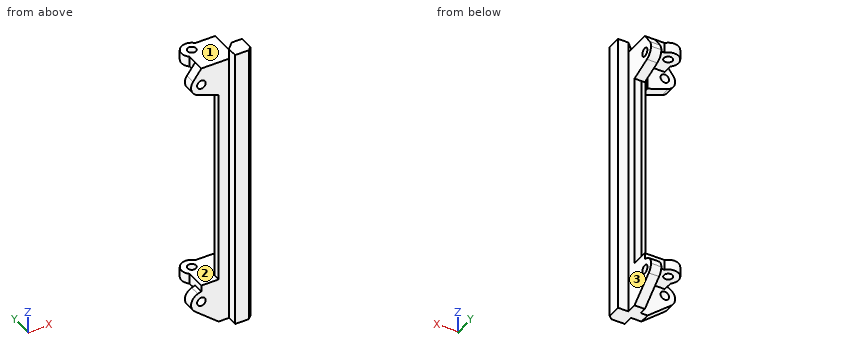
from build123d import *

# Parameters (mm, degrees)
F1_DEPTH  = 80
F2_R      = 1.25
F3_DEPTH  = 3
F4_DEPTH  = 3
F5_R      = 1.25
F6_DEPTH  = 3
F7_R      = 1.25
F8_DEPTH  = 3
F9_SIZE   = 1
F10_R     = 1.25
F10_W     = 3
F10_H     = 13
F11_DEPTH = 3
F12_W     = 3
F12_H     = 13
F12_R     = 1.25
F13_DEPTH = 3
F14_W     = 8
F14_H     = 3
F14_W_2   = 2
F15_DEPTH = 10
F17_DEPTH = 3
F16_R     = 1.25
F18_DEPTH = 25


with BuildPart() as f1:
    # F0 (on Top) → F1 (new body)
    with BuildSketch(Plane.XY):
        Polygon((40, 3), (40, 0), (45, 0), (45, 5), (42, 5), (42, 8), (40, 8), (40, 5), (37, 5), (37, 3), align=None)
    extrude(amount=F1_DEPTH)

    # F2 (on face) → F3 (join)
    with BuildSketch(Plane.XY.offset(80)):
        with BuildLine():
            Line((32, 3), (37, 3))
            Line((37, 3), (37, 5))
            Line((37, 5), (40, 5))
            Line((40, 5), (40, 8))
            Line((40, 8), (42, 8))
            Line((42, 8), (42, 13))
            Line((42, 13), (36.2360679775, 13))
            ThreePointArc((36.2360679775, 13), (36.8025170769, 12.0704662693), (37, 11))
            ThreePointArc((37, 11), (35.2247448714, 8.2613872125), (32, 8.7639320225))
            Line((32, 8.7639320225), (32, 3))
        make_face()
        with BuildLine():
            ThreePointArc((36.2360679775, 13), (31.8786796564, 13.1213203436), (32, 8.7639320225))
            ThreePointArc((32, 8.7639320225), (35.2247448714, 8.2613872125), (37, 11))
            ThreePointArc((37, 11), (36.8025170769, 12.0704662693), (36.2360679775, 13))
        make_face()
        with Locations((34, 11)):
            Circle(F2_R, mode=Mode.SUBTRACT)
    extrude(amount=-F3_DEPTH)

    # F2 (on face) → F4 (join)
    with BuildSketch(Plane.XY.offset(80)):
        Polygon((42, 5), (40, 3), (40, 0), (45, 0), (45, 5), align=None)
    extrude(amount=F4_DEPTH)

    # F5 (on face) → F6 (join)
    with BuildSketch(Plane.XZ.offset(-3)):
        with BuildLine():
            Line((32, 77), (32, 78))
            ThreePointArc((32, 78), (30.6583592135, 77.683281573), (29.6, 76.8))
            ThreePointArc((29.6, 76.8), (29.1245100257, 74.144688707), (30.97393957, 72.1809221376))
            ThreePointArc((30.97393957, 72.1809221376), (33.7207293091, 72.5425438671), (35, 75))
            ThreePointArc((35, 75), (34.8025170769, 76.0704662693), (34.2360679775, 77))
            Line((34.2360679775, 77), (32, 77))
        make_face()
        with Locations((32, 75)):
            Circle(F5_R, mode=Mode.SUBTRACT)
        with BuildLine():
            ThreePointArc((29.6, 76.8), (30.6583592135, 77.683281573), (32, 78))
            Line((32, 78), (32, 80))
            Line((32, 80), (29.6, 76.8))
        make_face()
        with BuildLine():
            Line((37, 77), (34.2360679775, 77))
            ThreePointArc((34.2360679775, 77), (34.8025170769, 76.0704662693), (35, 75))
            ThreePointArc((35, 75), (33.7207293091, 72.5425438671), (30.97393957, 72.1809221376))
            Line((30.97393957, 72.1809221376), (37, 69.9876155112))
            Line((37, 69.9876155112), (37, 77))
        make_face()
    extrude(amount=-F6_DEPTH)

    # F7 (on face) → F8 (join)
    with BuildSketch(Plane.YZ.offset(42)):
        with BuildLine():
            Line((8, 69.9876155112), (14.02606043, 72.1809221376))
            ThreePointArc((14.02606043, 72.1809221376), (10.5156676094, 73.3183066353), (10.7639320225, 77))
            Line((10.7639320225, 77), (8, 77))
            Line((8, 77), (8, 69.9876155112))
        make_face()
        with BuildLine():
            ThreePointArc((14.02606043, 72.1809221376), (15.4574561329, 73.2792706909), (16, 75))
            ThreePointArc((16, 75), (15.8460498942, 75.9486832981), (15.4, 76.8))
            ThreePointArc((15.4, 76.8), (14.3416407865, 77.683281573), (13, 78))
            Line((13, 78), (13, 77))
            Line((13, 77), (10.7639320225, 77))
            ThreePointArc((10.7639320225, 77), (10.5156676094, 73.3183066353), (14.02606043, 72.1809221376))
        make_face()
        with Locations((13, 75)):
            Circle(F7_R, mode=Mode.SUBTRACT)
        with BuildLine():
            ThreePointArc((13, 78), (14.3416407865, 77.683281573), (15.4, 76.8))
            Line((15.4, 76.8), (13, 80))
            Line((13, 80), (13, 78))
        make_face()
    extrude(amount=-F8_DEPTH)

    # F9
    f9_edges = [f1.edges().sort_by_distance(p)[0] for p in [
        (45, 0, 41.5),
    ]]
    chamfer(f9_edges, length=F9_SIZE)

    # F10 (on face) → F11 (join)
    with BuildSketch(Plane.XZ.offset(-3)):
        with BuildLine():
            ThreePointArc((30.0936794849, 5.6835496781), (33.2808275557, 5.2871637033), (35, 8))
            ThreePointArc((35, 8), (33.7229608507, 10.4558920796), (30.9790627288, 10.8209372712))
            ThreePointArc((30.9790627288, 10.8209372712), (29.0435836969, 8.5095121614), (30.0936794849, 5.6835496781))
        make_face()
        with Locations((32, 8)):
            Circle(F10_R, mode=Mode.SUBTRACT)
        with BuildLine():
            ThreePointArc((30.9790627288, 10.8209372712), (33.7229608507, 10.4558920796), (35, 8))
            ThreePointArc((35, 8), (33.2808275557, 5.2871637033), (30.0936794849, 5.6835496781))
            Line((30.0936794849, 5.6835496781), (37, 0))
            Line((37, 0), (37, 13))
            Line((37, 13), (30.9790627288, 10.8209372712))
        make_face()
        with Locations((38.5, 6.5)):
            Rectangle(F10_W, F10_H)
    extrude(amount=-F11_DEPTH)

    # F12 (on face) → F13 (join)
    with BuildSketch(Plane.YZ.offset(42)):
        with Locations((6.5, 6.5)):
            Rectangle(F12_W, F12_H)
        with BuildLine():
            ThreePointArc((14.9063205151, 5.6835496781), (10.0435836969, 7.4904878386), (14.0209372712, 10.8209372712))
            Line((14.0209372712, 10.8209372712), (8, 13))
            Line((8, 13), (8, 0))
            Line((8, 0), (14.9063205151, 5.6835496781))
        make_face()
        with BuildLine():
            ThreePointArc((14.9063205151, 5.6835496781), (15.7128362967, 6.7191724443), (16, 8))
            ThreePointArc((16, 8), (15.4558920796, 9.7229608507), (14.0209372712, 10.8209372712))
            ThreePointArc((14.0209372712, 10.8209372712), (10.0435836969, 7.4904878386), (14.9063205151, 5.6835496781))
        make_face()
        with Locations((13, 8)):
            Circle(F12_R, mode=Mode.SUBTRACT)
    extrude(amount=-F13_DEPTH)

    # F14 (on face) → F15 (join)
    with BuildSketch(Plane.XZ.offset(-3)):
        with Locations((36, 11.5)):
            Rectangle(F14_W, F14_H)
        with Locations((41, 11.5)):
            Rectangle(F14_W_2, F14_H)
    extrude(amount=-F15_DEPTH)

    # F16 (on face) → F17 (join)
    with BuildSketch(Plane.XY.offset(13)):
        with BuildLine():
            Line((32, 13), (36.2360679775, 13))
            ThreePointArc((36.2360679775, 13), (31.8786796564, 13.1213203436), (32, 8.7639320225))
            Line((32, 8.7639320225), (32, 13))
        make_face()
    extrude(amount=-F17_DEPTH)

    # F16 (on face) → F18 (cut)
    with BuildSketch(Plane.XY.offset(13)):
        with Locations((34, 11)):
            Circle(F16_R)
    extrude(amount=-F18_DEPTH, mode=Mode.SUBTRACT)


solid = f1.part
Could you check a few things on this model? Use its own coordinates, in mm. Face numbers are marked on the shaded views. Coordinates: 2 decimals unless noted, no trailing zeros. Write each loop counter-clockwise with the first axis right and the second up, starting at its lowest first coordinate (ties: lowest second). Pieces come first, ordered by that corner, then holes. Notation, with made-up numbers: M -36.75,-34 L 9.25,-34 A10 cw 9.25,-25 Z; hole C -26.75,47.25 d7. An arc over 180 degrees is marked long. One line per question, with ' | ' between items.
1) If we mould it in two halves opening along Z, with no side actions, what happens to the marked faces 1, 2 and 3? For each: released by +Z, released by -Z, zero draft, split by the parting line, or undercut.
Checks:
face 1: released by +Z | face 2: undercut | face 3: zero draft
2) For pin 1 Ø9 at (y, z) = (11.5, 76.5) entering from -X; pin 2 Ø3 at (y, z) = (7.5, 51) entering from -X; pin 3 Ø0.8 at (y, z) = (5.5, 73) entering from +X, each with a flat end and sliding along its axis, tell me the tip position at first contact or that it passes through.
Checks:
pin 1: x = 31 | pin 2: x = 40 | pin 3: x = 42
3) Imagine slicing it at A-A, the plane z = 37.5. Write out the boundary of the cut face in (x, y).
Checks:
outline: M 37,3 L 40,3 L 40,0 L 44,0 L 45,1 L 45,5 L 42,5 L 42,8 L 40,8 L 40,5 L 37,5 Z
4) I need wall thicknesses on probe 1 along Y at (x, z) = (34, 78.4); probe 2 along Z at (x, y) = (31.75, 12); probe 3 along Y at (x, z) = (40.55, 75). Which ranges of each line are inside material? Lowest first, please. Write a range as [from, to].
Checks:
probe 1: [3, 9.75], [12.25, 14] | probe 2: [10, 13], [77, 80] | probe 3: [0, 11.75], [14.25, 16]
5) Imagine slicing it at B-B, the plane y = 11. Write out the boundary of the cut face in (x, z), and give its area (3 significant figures).
Checks:
outline: M 31,10 L 32.75,10 L 32.75,13 L 31,13 Z; M 31,77 L 32.75,77 L 32.75,80 L 31,80 Z; M 35.25,10 L 39,10 L 39,2.47 L 42,2.47 L 42,13 L 35.25,13 Z; M 35.25,77 L 39,77 L 39,71.08 L 42,71.08 L 42,80 L 35.25,80 Z | area: 91.4 mm²
6) Imagine slicing it at C-C, the plane x = 34. Write out the boundary of the cut face in (y, z).
Checks:
outline: M 3,2.47 L 6,2.47 L 6,10 L 9.75,10 L 9.75,13 L 3,13 Z; M 3,71.08 L 6,71.08 L 6,77 L 9.75,77 L 9.75,80 L 3,80 Z; M 12.25,10 L 14,10 L 14,13 L 12.25,13 Z; M 12.25,77 L 14,77 L 14,80 L 12.25,80 Z
